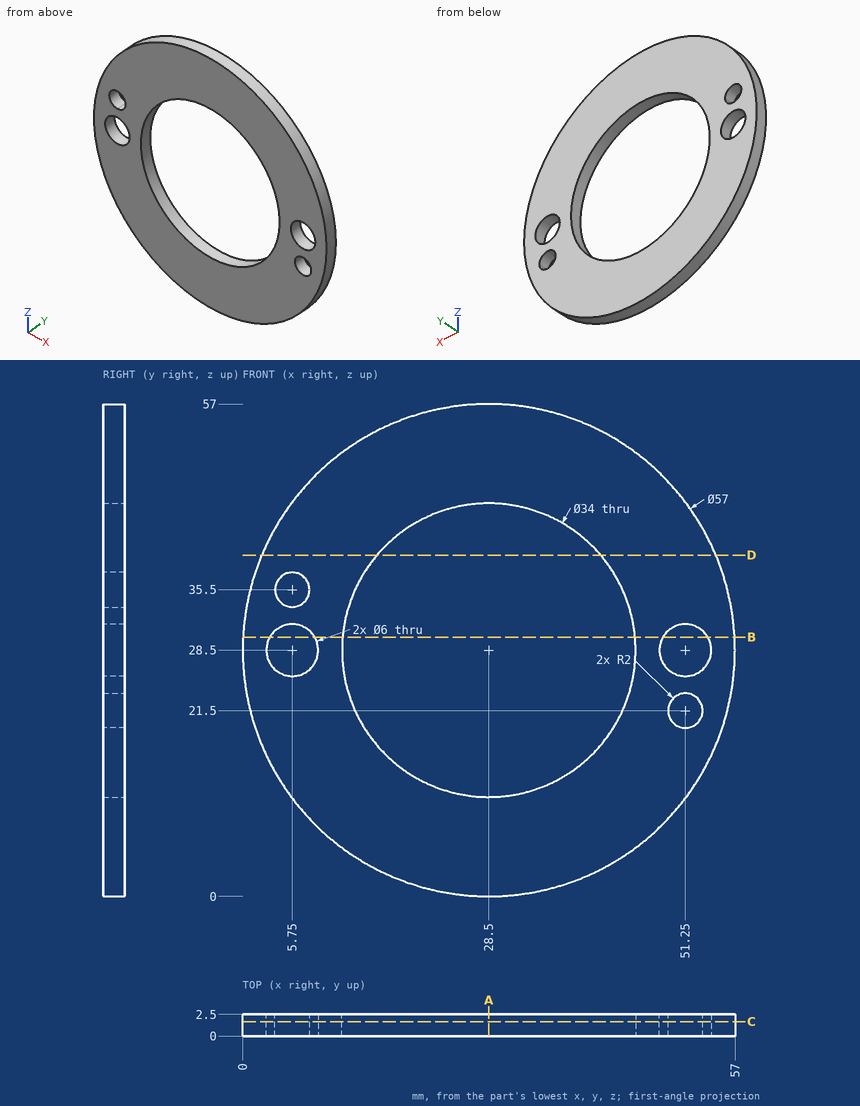
Input: dimensioned drawing with shaded views. Units: mm. Origin: part minimum x, y, z. Coordinates: 2 decimals unless noted, no trailing zeros. Loops run counter-clockwise (first coordinate to the right, second up) from the corner with the lowest first, then second, coordinate; pieces in that order, holes last. Notation, with made-up numbers: M 58,-18 L 67,-18 A20 ccw 67,-13 Z; hole C 37,-3.75 d5. An arc over 180 degrees is marked long. Use a Markdown table: item, result. Add a question column.
Q1. Section query C-C, the plane y = 1.65. Return loops of the section in (x, z), and give its area (3 significant figures).
Q2. Section query B-B, the plane z = 30. Return loops of the section in (x, y).
Q3. Material intervals for L1, parallel to Z at x = 5.75, y = 1.65; L2, parallel to Z at x = 49.5, y = 1.9; L3, parallel to X at y = 1.1, z = 13, sorted ascending.
Q4. First-contact query: pin 1 (7 mm diameter, centred on x = 51.25, z = 28.5, fed in from -Y); pin 2 (1.5 mm diameter, centred on y = 1, z = 10, fed in from +X); pin 3 (5.5 mm diameter, centred on x = 5.75, z = 28.5, fed in from +Y); pin 4 (1 mm diameter, centred on y = 2, z = 40, fed in from +X). Flat tips, straight axial feed; report the tip coordinate or a pass-through.
Q5. Section query D-D, the plane z = 39.5. Return loops of the section in (x, y).
Q6. Section query A-A, the plane x = 28.5. Return loops of the section in (y, z).
Result:
| question | item | result |
|---|---|---|
| 1 | outline | C 28.5,28.5 d57; hole C 5.75,28.5 d6; hole C 5.75,35.5 d4; hole C 28.5,28.5 d34; hole C 51.25,28.5 d6; hole C 51.25,21.5 d4 |
| 1 | area | 1,560 mm2 |
| 2 | outline | M 0.04,0 L 3.15,0 L 3.15,2.5 L 0.04,2.5 Z; M 8.35,0 L 11.57,0 L 11.57,2.5 L 8.35,2.5 Z; M 45.43,0 L 48.65,0 L 48.65,2.5 L 45.43,2.5 Z; M 53.85,0 L 56.96,0 L 56.96,2.5 L 53.85,2.5 Z |
| 3 | L1 | z = 11.33 to 25.5, 31.5 to 33.5, 37.5 to 45.67 |
| 3 | L2 | z = 9.23 to 20.53, 22.47 to 26.06, 30.94 to 47.77 |
| 3 | L3 | x = 4.58 to 21.52, 35.48 to 52.42 |
| 4 | pin 1 | stops at y = 0 |
| 4 | pin 2 | stops at x = 50.8 |
| 4 | pin 3 | passes through |
| 4 | pin 4 | stops at x = 54.79 |
| 5 | outline | M 2.21,0 L 15.54,0 L 15.54,2.5 L 2.21,2.5 Z; M 41.46,0 L 54.79,0 L 54.79,2.5 L 41.46,2.5 Z |
| 6 | outline | M 0,0 L 2.5,0 L 2.5,11.5 L 0,11.5 Z; M 0,45.5 L 2.5,45.5 L 2.5,57 L 0,57 Z |
